The listing builds one solid part. Answer for the finished solid, in the listing's coordinates (mm). Face numbers are marked on the shaded views. A direction names the side the tool comes from. Round coordinates to 2 decimals unless told otherwise and drop trailing zeros. Loops run counter-clockwise (first coordinate to the right, second up) from the corner with the lowest first, then second, coordinate; pieces in that order, holes last. Notation, with made-up numbers: (-20, -36) - (-9, -36) arc R22 ccw to (-9, -26) - close; hole circle Ø1 at (-27, -19.5). An arc over 180 degrees is marked (long way). One line per question, with ' | ' between items. Start each with the question number.
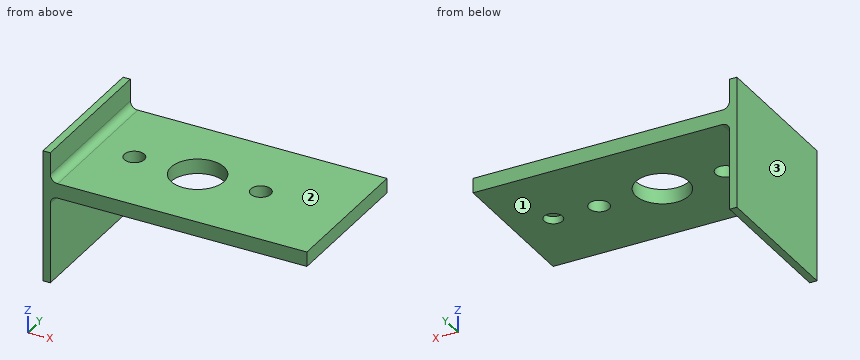
Autodesk Inventor part; units mm, degrees
ref_plane "YZ Plane" through (0, 0, 0) normal (1, 0, 0) x (0, 1, 0)
ref_plane "XZ Plane" through (0, 0, 0) normal (0, 1, 0) x (-1, 0, 0)
ref_plane "XY Plane" through (0, 0, 0) normal (0, 0, 1) x (1, 0, 0)
sketch "Sketch1" plane through (0, 0, 0) normal (0, 0, 1) x (1, 0, 0)
  line L0 (-12.9399, 8.8675) -> (22.0601, 8.8675)
  line L1 (22.0601, 8.8675) -> (22.0601, -11.1325)
  line L2 (22.0601, -11.1325) -> (-12.9399, -11.1325)
  line L3 (-12.9399, -11.1325) -> (-12.9399, 8.8675)
  circle A0 centre (-6.9399, -1.1325) radius 1.375
  circle A1 centre (10.3101, -1.1325) radius 1.375
  circle A2 centre (1.6851, -1.1325) radius 3.625
  circle A3 centre (16.5601, -1.1325) radius 1.25
  point P0 (0, 0)
  dimension "d0" = 20
  dimension "d1" = 35
  dimension "d2" = 7.25
  dimension "d3" = 2.75
  dimension "d4" = 2.75
  dimension "d5" = 8.625
  dimension "d6" = 0
  dimension "d7" = 8.625
  dimension "d8" = 0
  dimension "d9" = 6
  dimension "d10" = 10
  dimension "d20" = 2.5
  dimension "d21" = 14.875
  dimension "d24" = 6.25
extrude "Extrusion1" add sketch "Sketch1" along normal blind 2 contours L0 L1 L2 L3 | A3
sketch "Sketch2" plane through (-12.9399, -11.1325, 0) normal (-1, 0, 0) x (0, 0, 1)
  line L0 (-12, 20) -> (6, 20)
  line L1 (6, 20) -> (6, 0)
  line L2 (6, 0) -> (-12, 0)
  line L3 (-12, 0) -> (-12, 20)
  line L4 (0, 0) -> (0, 20)
  line L5 (2, 20) -> (2, 0)
  point P0 (0, 11.1325)
  dimension "d13" = 12
  dimension "d14" = 4
  dimension "d15" = 0
  dimension "d16" = 0
extrude "Extrusion2" add sketch "Sketch2" along normal blind 1
fillet "Fillet1" radius 1 2 edges at (-12.9399, -1.1325, 2) (-12.9399, -1.1325, 0)
extrude "Extrusion3" cut sketch "Sketch1" along normal blind 1 contours A3
equation "\"d7\" = d5"
properties part number "tac switch test"
(1) A tool of negligible diameter and unlimited length cuts with its end or side. For the marked faces 1, 2 and 3, from which of +Z, -Z, +X, -X, +Y, -Y can it reach the whole face along a straight path? Write none if from no direction.
(2) Find section B-B on y = -4. Write down the section's boundary in (x, z).
(3) Find section A-A on x = -1.5. Write down the section's boundary in (y, z), plus the area to 3 significant figures.
(4) Find section C-C on y = -6. Write down the section's boundary in (x, z).
(5) Each of these flat-tipped pins is pushed along its axis until it touches: P1, Ø1.2, axis at x = 17, y = -0.5, coming from the -Z side; P2, Ø2, axis at x = 16.56, y = -1.13, coming from the -Z side; P3, Ø0.9, axis at y = -1.5, z = 4.5, coming from the +X side. Where does it stop, or does it pass through?
(6) Consider L1, parallel to Z at x = 2, y = -10; L2, parallel to X at y = -3.75, z = -1; L3, parallel to X at y = -1.5, z = 0.5. Determine where each line is inside the solid, lowest interval first.
(7) Find section D-D on x = 13.5. Write down the section's boundary in (y, z), plus the area to 3 significant figures.
Answer below:
1) face 1: -Z, +X, +Y, -Y | face 2: +Z, +X, +Y, -Y | face 3: +Z, -Z, -X, +Y, -Y
2) outline: (-13.94, -12) - (-12.94, -12) - (-12.94, -1) arc R1 cw to (-11.94, 0) - (-0.53, 0) - (-0.53, 2) - (-11.94, 2) arc R1 cw to (-12.94, 3) - (-12.94, 6) - (-13.94, 6) - close; (3.9, 0) - (22.06, 0) - (22.06, 2) - (3.9, 2) - close
3) outline: (-11.13, 0) - (-2.86, 0) - (-2.86, 2) - (-11.13, 2) - close; (0.6, 0) - (8.87, 0) - (8.87, 2) - (0.6, 2) - close | area: 33.1 mm2
4) outline: (-13.94, -12) - (-12.94, -12) - (-12.94, -1) arc R1 cw to (-11.94, 0) - (22.06, 0) - (22.06, 2) - (-11.94, 2) arc R1 cw to (-12.94, 3) - (-12.94, 6) - (-13.94, 6) - close
5) P1: z = 0 | P2: z = 1 | P3: x = -12.94
6) L1: 0 to 2 | L2: -13.94 to -12.94 | L3: -13.94 to -8.26, -5.61 to -1.92, 5.29 to 8.99, 11.64 to 15.37, 17.75 to 22.06
7) outline: (-11.13, 0) - (8.87, 0) - (8.87, 2) - (-11.13, 2) - close | area: 40.0 mm2
